Geometry check sheet. Reference: the model listing, model coordinates, mm. A direction names the side the tool comes from. Give positions to 0.01 mm unless a question says otherwise; leave off trailing zeros. Loops run counter-clockwise (first coordinate to the right, second up) from the corner with the lowest first, then second, coordinate; pieces in that order, holes last. Notation, with made-up numbers: (-3, -35.75) -> (10, -35.75) arc R18 cw to (10, -27.75) -> close; hole circle Ø2 at (-13, -13.75). An arc over 180 degrees is marked (long way). One line per question, with ' | ' between items.
from build123d import *

# Parameters (mm, degrees)
F0_R     = 1.7
F1_DEPTH = 4
F2_DEPTH = 20
F3_R     = 1.5
F4_DEPTH = 10
F5_SIZE  = 1


with BuildPart() as f1:
    # F0 (on Top) → F1 (new body)
    with BuildSketch(Plane.XY):
        Polygon((-4, 3.448833), (-8, 3.448833), (-8, -3.551167), (0.5, -3.551167), (0.5, 3.448833), align=None)
        with Locations((-4, 0)):
            Circle(F0_R, mode=Mode.SUBTRACT)
    extrude(amount=F1_DEPTH)

    # F0 (on Top) → F2 (join)
    with BuildSketch(Plane.XY):
        Polygon((-8, -3.551167), (-8, 3.448833), (-28, 3.448833), (-28, -3.551167), (-28, -6.551167), (-8, -6.551167), align=None)
    extrude(amount=F2_DEPTH)

    # F3 (on face) → F4 (cut, through all)
    with BuildSketch(Plane.XZ.offset(6.551167)):
        with Locations((-13, 14)):
            Circle(F3_R)
        with Locations((-23, 14)):
            Circle(F3_R)
    extrude(amount=-F4_DEPTH, mode=Mode.SUBTRACT)

    # F5
    f5_edges = [f1.edges().sort_by_distance(p)[0] for p in [
        (-8, -6.551167, 10),
        (-28, -6.551167, 10),
        (-8, 3.448833, 12),
        (-28, 3.448833, 10),
        (0.5, -3.551167, 2),
        (-8, -3.551167, 2),
        (0.5, 3.448833, 2),
    ]]
    chamfer(f5_edges, length=F5_SIZE)


solid = f1.part
Item 1: Release check for a two-part mould opening along Z. For faces 1 (the face through (-2.43, -0.65, 1.97)), 2 (the face through (-14.5, -1.62, 14.07)), 3 (the face through (-24.5, -1.62, 14.07)), 4 (the face through (-18, -1, 20)) record: pulls with the +Z half, pulls with the -Z half, needs draft (parallel to the pull), parting line crosses it, or undercut.
Result:
face 1: needs draft | face 2: undercut | face 3: undercut | face 4: pulls with the +Z half
Item 2: Sectioned sample at A-A (x = -4). Record the cut outline in (y, z).
Result:
outline: (-3.55, 0) -> (-1.7, 0) -> (-1.7, 4) -> (-3.55, 4) -> close; (1.7, 0) -> (3.45, 0) -> (3.45, 4) -> (1.7, 4) -> close
Item 3: Depth check by flat-ended pin: pin 1 Ø4.5 at (x, y) = (-4, 0) entering from +Z; pin 2 Ø4.5 at (x, z) = (-4, 2) entering from -Y. Enter the tip coordinate at first touch or a pass-through.
Result:
pin 1: z = 4 | pin 2: y = -3.55
Item 4: Sectioned sample at D-D (x = -13). Record the cut outline in (y, z), plus the area to 3 significant figures.
Result:
outline: (-6.55, 0) -> (3.45, 0) -> (3.45, 12.5) -> (-6.55, 12.5) -> close; (-6.55, 15.5) -> (3.45, 15.5) -> (3.45, 20) -> (-6.55, 20) -> close | area: 170 mm2
Item 5: Sectioned sample at B-B (y = 0). Record the cut outline in (x, z), plus the area to 3 significant figures.
Result:
outline: (-28, 0) -> (-5.7, 0) -> (-5.7, 4) -> (-8, 4) -> (-8, 20) -> (-28, 20) -> close; (-2.3, 0) -> (0.5, 0) -> (0.5, 4) -> (-2.3, 4) -> close; hole circle Ø3 at (-23, 14); hole circle Ø3 at (-13, 14) | area: 406 mm2
Item 6: Scan lines: probe 1 along Z at (x, y) = (-23, -0.5); probe 2 along Y at (x, z) = (-4, 2.4); probe 3 along X at (y, z) = (-2.25, 13.25). Record each from-to range of solid material in increasing order.
Result:
probe 1: 0 to 12.5, 15.5 to 20 | probe 2: -3.55 to -1.7, 1.7 to 3.45 | probe 3: -28 to -24.3, -21.7 to -14.3, -11.7 to -8
Item 7: Set-up check for faces 5 (the face through (0.01, 2.94, 1.97)), 6 (the face through (-8.49, 2.94, 11.89)), 7 (the face through (-4, -3.551, 2)): record each of +Z, -Z, +X, -X, +Y, -Y from which the full face is reachable in a straight line by a thin tool's end or side.
Result:
face 5: +Z, -Z, +X, +Y | face 6: +Z, +X, +Y | face 7: +Z, -Z, +X, -Y
Item 8: Sectioned sample at C-C (z = 3). Record the cut outline in (x, y).
Result:
outline: (-28, -5.55) -> (-27, -6.55) -> (-9, -6.55) -> (-8, -5.55) -> (-8, -4.55) -> (-7, -3.55) -> (-0.5, -3.55) -> (0.5, -2.55) -> (0.5, 2.45) -> (-0.5, 3.45) -> (-27, 3.45) -> (-28, 2.45) -> close; hole circle Ø3.4 at (-4, 0)
